Here's how the part is built. I have some questions about the finished solid (model axes, mm). Face numbers are marked on the shaded views. A direction names the side the tool comes from. Give positions to 0.01 mm unless a question says otherwise; leave off trailing zeros. Loops run counter-clockwise (first coordinate to the right, second up) from the corner with the lowest first, then second, coordinate; pieces in that order, holes last.
Q1. For the marked faces 1, 2, 3 and 4, which set-ups out of +Z, -Z, +X, -X, +Y, -Y let a thin tool reach every point of the face, with its end or its side?
Q2. I need wall thicknesses on line 1 (X direction, y = 132, z = 47.5); line 2 (X direction, y = 80, z = -17); line 3 (Z direction, x = -217, y = 187). Which ranges of each line are inside material? Lowest first, please.
Q3. If we section it at B-B (z = -40.5): Please give me the cut outline in (x, y).
Q4. If we section it at C-C (y = 182): Please give me the cut outline in (x, z).
Q5. Will this pin go through, and if not, where does the flat tip stop? P1, Ø12, axis at y = 148.5, z = -43.5, coming from the -X side.
Q6. If we section it at D-D (y = 45.5): Please give me the cut outline in (x, z), plus the area to 3 significant figures.
Q7. We'd pull the mould along Z, two halves only. Please class the marked faces 5 and 6: +Z half, -Z half, draft (parallel to the pull), parting line (faces both ways), or undercut.
Q8. If we section it at A-A (x = 448): Please give me the cut outline in (y, z).
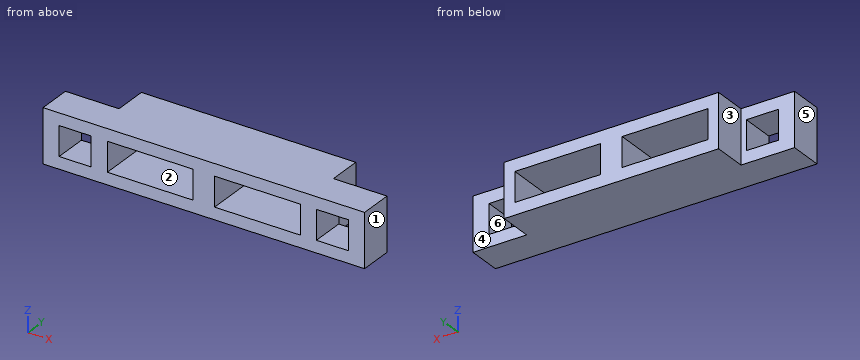
from build123d import *

# Parameters (mm, degrees)
SKETCH_1_W          = 1200
SKETCH_1_H          = 200
SKETCH_1_W_2        = 120
SKETCH_1_H_2        = 110
SKETCH_1_W_3        = 320
EXTRUDE_1_DEPTH     = 250
SKETCH_2_W          = 200
SKETCH_2_H          = 125
CUT_EXTRUDE_1_DEPTH = 201


with BuildPart() as part:
    # Эскиз1 → Бобышка-Вытянуть1 (new body)
    with BuildSketch(Plane(origin=(0, 0, 0), x_dir=(1, 0, 0), z_dir=(0, 1, 0))):
        Rectangle(SKETCH_1_W, SKETCH_1_H)
        with Locations((-480, 0)):
            Rectangle(SKETCH_1_W_2, SKETCH_1_H_2, mode=Mode.SUBTRACT)
        with Locations((-200, 0)):
            Rectangle(SKETCH_1_W_3, SKETCH_1_H_2, mode=Mode.SUBTRACT)
        with Locations((200, 0)):
            Rectangle(SKETCH_1_W_3, SKETCH_1_H_2, mode=Mode.SUBTRACT)
        with Locations((480, 0)):
            Rectangle(SKETCH_1_W_2, SKETCH_1_H_2, mode=Mode.SUBTRACT)
    extrude(amount=EXTRUDE_1_DEPTH)

    # Эскиз2 → Вырез-Вытянуть1 (cut, through all)
    with BuildSketch(Plane.XY.offset(100)):
        with Locations((-500, 187.5)):
            Rectangle(SKETCH_2_W, SKETCH_2_H)
        with Locations((500, 187.5)):
            Rectangle(SKETCH_2_W, SKETCH_2_H)
    extrude(amount=-CUT_EXTRUDE_1_DEPTH, mode=Mode.SUBTRACT)


solid = part.part
Check sheet entries:
1. face 1: +Z, -Z, +X, +Y, -Y
1. face 2: +Y, -Y
1. face 3: +Z, -Z, -X, +Y
1. face 4: +Z, -Z, +X, +Y
2. line 1: x = -400 to -360, -40 to 40, 360 to 400
2. line 2: x = -600 to -540, -420 to -360, -40 to 40, 360 to 420, 540 to 600
2. line 3: z = -100 to -55, 55 to 100
3. outline: (-600, 0) - (-540, 0) - (-540, 125) - (-600, 125) - close; (-420, 0) - (-360, 0) - (-360, 250) - (-400, 250) - (-400, 125) - (-420, 125) - close; (-40, 0) - (40, 0) - (40, 250) - (-40, 250) - close; (360, 0) - (420, 0) - (420, 125) - (400, 125) - (400, 250) - (360, 250) - close; (540, 0) - (600, 0) - (600, 125) - (540, 125) - close
4. outline: (-400, -100) - (400, -100) - (400, 100) - (-400, 100) - close; hole (-360, -55) - (-40, -55) - (-40, 55) - (-360, 55) - close; hole (40, -55) - (360, -55) - (360, 55) - (40, 55) - close
5. P1: stops at x = -400
6. outline: (-600, -100) - (600, -100) - (600, 100) - (-600, 100) - close; hole (-540, -55) - (-420, -55) - (-420, 55) - (-540, 55) - close; hole (-360, -55) - (-40, -55) - (-40, 55) - (-360, 55) - close; hole (40, -55) - (360, -55) - (360, 55) - (40, 55) - close; hole (420, -55) - (540, -55) - (540, 55) - (420, 55) - close
6. area: 143,000 mm2
7. face 5: draft
7. face 6: undercut
8. outline: (0, -100) - (125, -100) - (125, -55) - (0, -55) - close; (0, 55) - (125, 55) - (125, 100) - (0, 100) - close
